Verification items for this drawing (mm, ordinates from the low corner). Give positions to 0.01 mm unless a question says otherwise; leave off trailing zeros. Loops run counter-clockwise (first coordinate to the right, second up) from the corner with the lowest first, then second, coordinate; pieces in that order, holes last. Notation, with made-up numbers: M 50,85 L 98,85 A4 cw 98,91 Z; hole C -9,4.25 d10. An arc over 180 degrees is marked long. Use a Markdown table: item, result.
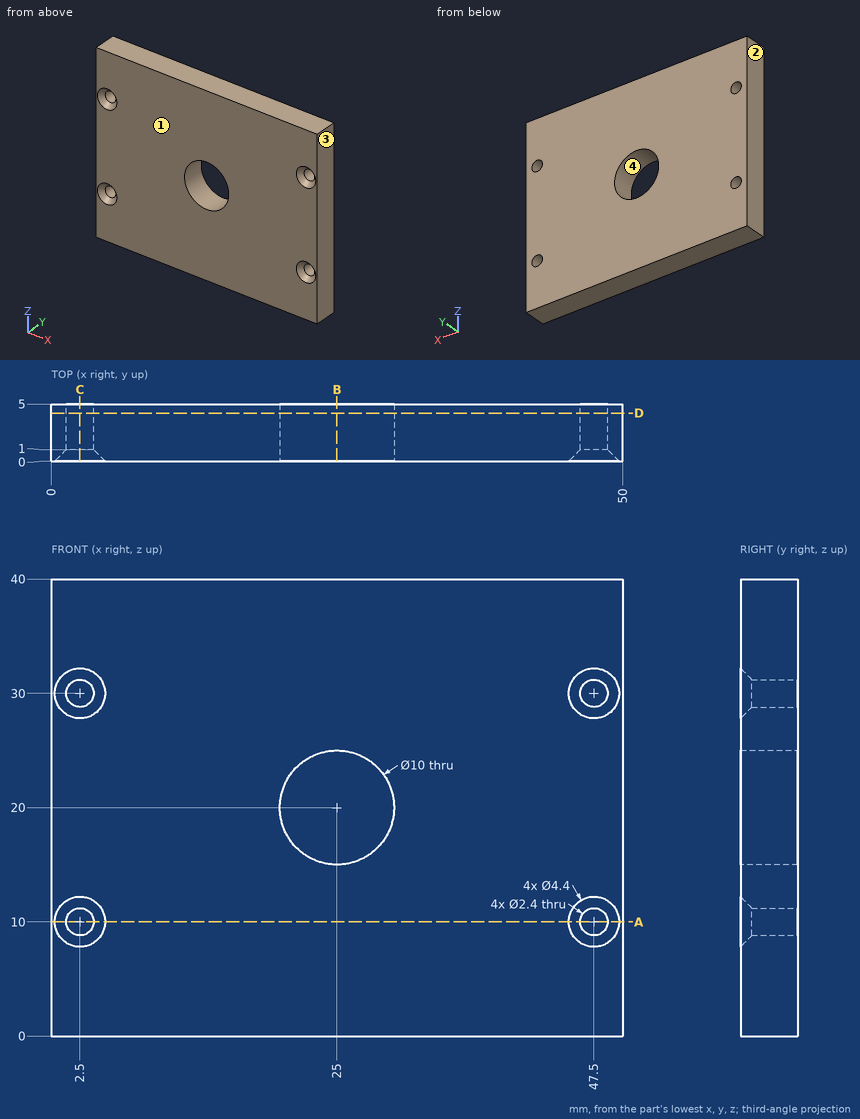
(1) Cross-section at A-A on z = 10. Record the cut outline in (x, y), then the cut area to 3 significant figures.
Results below:
| item | result |
|---|---|
| outline | M 0,0 L 0.3,0 L 1.3,1 L 1.3,5 L 0,5 Z; M 3.7,1 L 4.7,0 L 45.3,0 L 46.3,1 L 46.3,5 L 3.7,5 Z; M 48.7,1 L 49.7,0 L 50,0 L 50,5 L 48.7,5 Z |
| area | 224 mm^2 |
(2) Material ranges on line 1 (Z direction, x = 2.5, y = 2.2); line 2 (X direction, y = 3.8, z = 20); line 3 (X direction, y = 3.65, z = 30), recorded low to high.
Results below:
| item | result |
|---|---|
| line 1 | 0 to 8.8, 11.2 to 28.8, 31.2 to 40 |
| line 2 | 0 to 20, 30 to 50 |
| line 3 | 0 to 1.3, 3.7 to 46.3, 48.7 to 50 |
(3) Cross-section at B-B on x = 25. Record the cut outline in (y, z), then the cut area to 3 significant figures.
Results below:
| item | result |
|---|---|
| outline | M 0,0 L 5,0 L 5,15 L 0,15 Z; M 0,25 L 5,25 L 5,40 L 0,40 Z |
| area | 150 mm^2 |
(4) Cross-section at D-D on y = 4.2. Record the cut outline in (x, z), then the cut area to 3 significant figures.
Results below:
| item | result |
|---|---|
| outline | M 0,0 L 50,0 L 50,40 L 0,40 Z; hole C 2.5,10 d2.4; hole C 2.5,30 d2.4; hole C 25,20 d10; hole C 47.5,10 d2.4; hole C 47.5,30 d2.4 |
| area | 1,900 mm^2 |
(5) Cross-section at C-C on x = 2.5. Record the cut outline in (y, z).
Results below:
| item | result |
|---|---|
| outline | M 0,0 L 5,0 L 5,8.8 L 1,8.8 L 0,7.8 Z; M 0,12.2 L 1,11.2 L 5,11.2 L 5,28.8 L 1,28.8 L 0,27.8 Z; M 0,32.2 L 1,31.2 L 5,31.2 L 5,40 L 0,40 Z |
(6) Gauge pin test, flat ends, axial feed: P1, Ø4, axis at x = 47.5, z = 10, coming from the -Y side; P2, Ø3, axis at x = 47.5, z = 30, coming from the -Y side. Record the tip position at first contact, or that the pin passes through.
Results below:
| item | result |
|---|---|
| P1 | y = 0.2 |
| P2 | y = 0.7 |
(7) Draft check along X on the marked faces 1, 2, 3 and 4. Enter one of: +X half, -X half, draft (parallel to the pull), parting line (faces both ways), or undercut.
Results below:
| item | result |
|---|---|
| face 1 | draft |
| face 2 | -X half |
| face 3 | +X half |
| face 4 | undercut |
